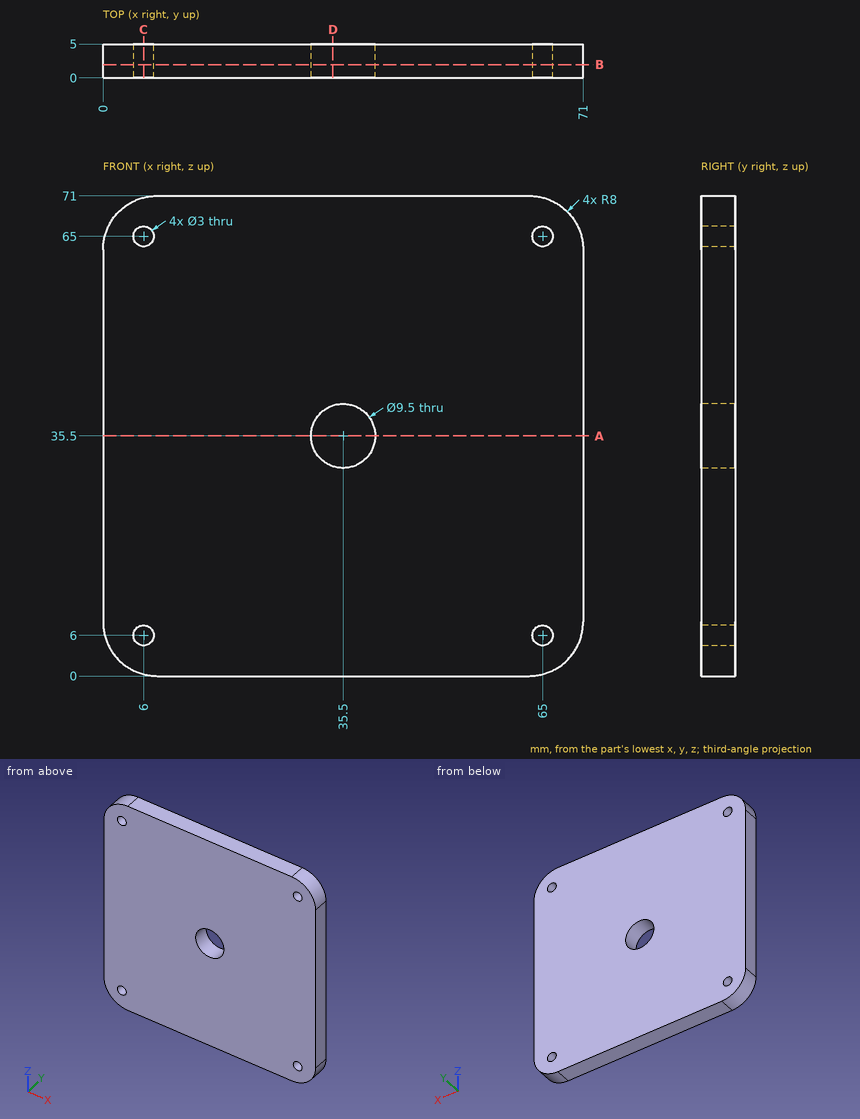
Can you work these out from the drawing? Everything is in mm from the part's minimum corner. Round coordinates to 2 decimals unless told otherwise and drop trailing zeros. Order: outer loops, then holes, each group sorted by start corner. A loop starts at its lowest first (then second) coordinate and runs counter-clockwise, first axis right, second up. Notation, with made-up numbers: (56, 49.5) -> (73, 49.5) arc R30 ccw to (73, 73.5) -> close; hole circle Ø2 at (-28, -5). An arc over 180 degrees is marked (long way). Return JSON: item names as keys, results as strings. Group by question number.
1. I need wall thicknesses on line 1 (X direction, y = 3.8, z = 64); line 2 (X direction, y = 2.3, z = 6); line 3 (Z direction, x = 35.5, y = 1.9). Which ranges of each line are inside material? Lowest first, please. Write a range as [from, to].
2. Will this pin go through, and if not, where does the flat tip stop? pin 1 (5.5 mm diameter, centred on x = 35.5, z = 35.5, fed in from +Y).
3. If we section it at B-B, the plane y = 1.95: Write out the boundary of the cut face in (x, z).
4. If we section it at D-D, the plane x = 34: Write out the boundary of the cut face in (y, z), then the cut area to 3 significant figures.
5. If we section it at A-A, the plane z = 35.5: Write out the boundary of the cut face in (x, y), then the cut area to 4 significant figures.
6. If we section it at C-C, the plane x = 6: Write out the boundary of the cut face in (y, z).
Output values:
{
 "1": {"line 1": "[0.06, 4.88], [7.12, 63.88], [66.12, 70.94]", "line 2": "[0.25, 4.5], [7.5, 63.5], [66.5, 70.75]", "line 3": "[0, 30.75], [40.25, 71]"},
 "2": {"pin 1": "through"},
 "3": {"outline": "(0, 8) arc R8 ccw to (8, 0) -> (63, 0) arc R8 ccw to (71, 8) -> (71, 63) arc R8 ccw to (63, 71) -> (8, 71) arc R8 ccw to (0, 63) -> close; hole circle Ø3 at (6, 6); hole circle Ø3 at (6, 65); hole circle Ø9.5 at (35.5, 35.5); hole circle Ø3 at (65, 6); hole circle Ø3 at (65, 65)"},
 "4": {"outline": "(0, 0) -> (5, 0) -> (5, 30.99) -> (0, 30.99) -> close; (0, 40.01) -> (5, 40.01) -> (5, 71) -> (0, 71) -> close", "area": "310 mm²"},
 "5": {"outline": "(0, 0) -> (30.75, 0) -> (30.75, 5) -> (0, 5) -> close; (40.25, 0) -> (71, 0) -> (71, 5) -> (40.25, 5) -> close", "area": "307.5 mm²"},
 "6": {"outline": "(0, 0.25) -> (5, 0.25) -> (5, 4.5) -> (0, 4.5) -> close; (0, 7.5) -> (5, 7.5) -> (5, 63.5) -> (0, 63.5) -> close; (0, 66.5) -> (5, 66.5) -> (5, 70.75) -> (0, 70.75) -> close"}
}
